```python
from build123d import *

# Parameters (mm, degrees)
SKETCH1_R           = 2.55
BOSS_EXTRUDE2_DEPTH = 10
SKETCH2_R           = 2.55
BOSS_EXTRUDE3_DEPTH = 2


with BuildPart() as part:
    # Sketch1 → Boss-Extrude2 (new body)
    with BuildSketch(Plane.XY):
        with BuildLine():
            ThreePointArc((18.024150889, 186.79103775), (10.644862344, 190.724335457), (2.347067513, 191.759386777))
            ThreePointArc((2.347067513, 191.759386777), (0, 191.690468331), (-2.347067513, 191.759386777))
            ThreePointArc((-2.347067513, 191.759386777), (-10.644862344, 190.724335457), (-18.024150889, 186.79103775))
            ThreePointArc((-18.024150889, 186.79103775), (-28.284271247, 194.215728749), (-35.708962247, 204.475849108))
            ThreePointArc((-35.708962247, 204.475849108), (-31.77566454, 211.855137653), (-30.74061322, 220.152932484))
            ThreePointArc((-30.74061322, 220.152932484), (-30.809531665, 222.499999997), (-30.74061322, 224.84706751))
            ThreePointArc((-30.74061322, 224.84706751), (-31.77566454, 233.14486234), (-35.708962247, 240.524150885))
            ThreePointArc((-35.708962247, 240.524150885), (-28.284271247, 250.784271244), (-18.024150889, 258.208962244))
            ThreePointArc((-18.024150889, 258.208962244), (-10.644862344, 254.275664537), (-2.347067513, 253.240613217))
            ThreePointArc((-2.347067513, 253.240613217), (0, 253.309531662), (2.347067513, 253.240613217))
            ThreePointArc((2.347067513, 253.240613217), (10.644862344, 254.275664537), (18.024150889, 258.208962244))
            ThreePointArc((18.024150889, 258.208962244), (28.284271247, 250.784271244), (35.708962247, 240.524150885))
            ThreePointArc((35.708962247, 240.524150885), (31.77566454, 233.14486234), (30.74061322, 224.84706751))
            ThreePointArc((30.74061322, 224.84706751), (30.809531665, 222.499999997), (30.74061322, 220.152932484))
            ThreePointArc((30.74061322, 220.152932484), (31.77566454, 211.855137653), (35.708962247, 204.475849108))
            ThreePointArc((35.708962247, 204.475849108), (28.284271247, 194.215728749), (18.024150889, 186.79103775))
        make_face()
        with Locations((-22.627416998, 245.127416995)):
            Circle(SKETCH1_R, mode=Mode.SUBTRACT)
        with Locations((-22.627416998, 199.872582999)):
            Circle(SKETCH1_R, mode=Mode.SUBTRACT)
        with Locations((22.627416998, 199.872582999)):
            Circle(SKETCH1_R, mode=Mode.SUBTRACT)
        with Locations((22.627416998, 245.127416995)):
            Circle(SKETCH1_R, mode=Mode.SUBTRACT)
        with BuildLine():
            Line((-15, 218.499999997), (-15, 199.25))
            Line((-15, 199.25), (15, 199.25))
            Line((15, 199.25), (15, 218.499999997))
            ThreePointArc((15, 218.499999997), (19, 222.499999997), (15, 226.499999997))
            Line((15, 226.499999997), (15, 245.749999994))
            Line((15, 245.749999994), (-15, 245.749999994))
            Line((-15, 245.749999994), (-15, 226.499999997))
            ThreePointArc((-15, 226.499999997), (-19, 222.499999997), (-15, 218.499999997))
        make_face(mode=Mode.SUBTRACT)
    extrude(amount=BOSS_EXTRUDE2_DEPTH)

    # Sketch2 → Boss-Extrude3 (add)
    with BuildSketch(Plane.XY.offset(10)):
        with BuildLine():
            ThreePointArc((18.024150889, 186.79103775), (28.284271247, 194.215728749), (35.708962247, 204.475849108))
            ThreePointArc((35.708962247, 204.475849108), (31.77566454, 211.855137653), (30.74061322, 220.152932484))
            ThreePointArc((30.74061322, 220.152932484), (30.809531665, 222.499999997), (30.74061322, 224.84706751))
            ThreePointArc((30.74061322, 224.84706751), (31.77566454, 233.14486234), (35.708962247, 240.524150885))
            ThreePointArc((35.708962247, 240.524150885), (28.284271247, 250.784271244), (18.024150889, 258.208962244))
            ThreePointArc((18.024150889, 258.208962244), (10.644862344, 254.275664537), (2.347067513, 253.240613217))
            ThreePointArc((2.347067513, 253.240613217), (0, 253.309531662), (-2.347067513, 253.240613217))
            ThreePointArc((-2.347067513, 253.240613217), (-10.644862344, 254.275664537), (-18.024150889, 258.208962244))
            ThreePointArc((-18.024150889, 258.208962244), (-28.284271247, 250.784271244), (-35.708962247, 240.524150885))
            ThreePointArc((-35.708962247, 240.524150885), (-31.77566454, 233.14486234), (-30.74061322, 224.84706751))
            ThreePointArc((-30.74061322, 224.84706751), (-30.809531665, 222.499999997), (-30.74061322, 220.152932484))
            ThreePointArc((-30.74061322, 220.152932484), (-31.77566454, 211.855137653), (-35.708962247, 204.475849108))
            ThreePointArc((-35.708962247, 204.475849108), (-28.284271247, 194.215728749), (-18.024150889, 186.79103775))
            ThreePointArc((-18.024150889, 186.79103775), (-10.644862344, 190.724335457), (-2.347067513, 191.759386777))
            ThreePointArc((-2.347067513, 191.759386777), (0, 191.690468331), (2.347067513, 191.759386777))
            ThreePointArc((2.347067513, 191.759386777), (10.644862344, 190.724335457), (18.024150889, 186.79103775))
        make_face()
        with Locations((-22.627416998, 245.127416995)):
            Circle(SKETCH2_R, mode=Mode.SUBTRACT)
        with Locations((-22.627416998, 199.872582999)):
            Circle(SKETCH2_R, mode=Mode.SUBTRACT)
        with Locations((22.627416998, 199.872582999)):
            Circle(SKETCH2_R, mode=Mode.SUBTRACT)
        with Locations((22.627416998, 245.127416995)):
            Circle(SKETCH2_R, mode=Mode.SUBTRACT)
        with BuildLine():
            Line((-15, 245.749999994), (-15, 226.499999997))
            ThreePointArc((-15, 226.499999997), (-19, 222.499999997), (-15, 218.499999997))
            Line((-15, 218.499999997), (15, 218.499999997))
            ThreePointArc((15, 218.499999997), (19, 222.499999997), (15, 226.499999997))
            Line((15, 226.499999997), (15, 245.749999994))
            Line((15, 245.749999994), (-15, 245.749999994))
        make_face(mode=Mode.SUBTRACT)
    extrude(amount=BOSS_EXTRUDE3_DEPTH)


solid = part.part
```
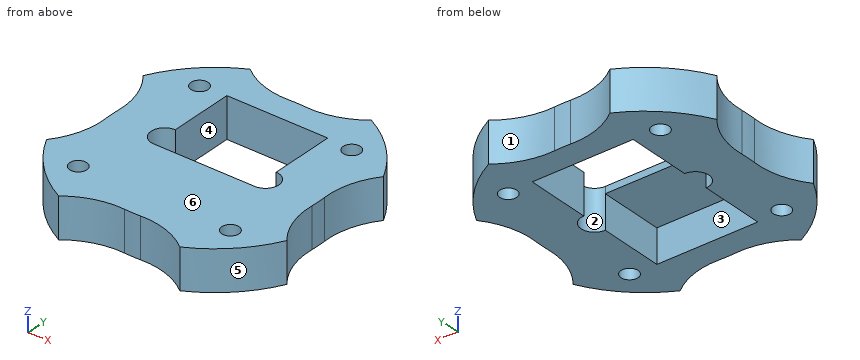
Input: part model. Units: mm. Frame: model coordinates. Face numbers are marked on the shaded views. A direction names the side the tool comes from. Coordinates: 2 decimals unless noted, no trailing zeros. Write each loop counter-clockwise with the first axis right and the second up, starting at its lowest first coordinate (ties: lowest second). Pieces come first, ordered by that corner, then holes. Notation, with made-up numbers: (31.25, -0.5) -> (63.25, -0.5) arc R32 cw to (63.25, 34.5) -> close; hole circle Ø9 at (80.25, 75.5). An arc over 180 degrees is marked (long way). Answer as a JSON object with one key per item and string values.
1. Section B-B on x = -8.5. Return the cut outline in (y, z), then the cut area to 3 significant figures.
Result set:
{"outline": "(191.29, 0) -> (199.25, 0) -> (199.25, 10) -> (218.5, 10) -> (218.5, 12) -> (191.29, 12) -> close; (245.75, 0) -> (253.71, 0) -> (253.71, 12) -> (245.75, 12) -> close", "area": "229 mm2"}
2. Mould query, pull axis X, two halves, no side actions, for the marked faces 4, 5 and 6. Classes: released by +X, released by -X, zero draft, split by the parting line, or undercut.
Result set:
{"face 4": "undercut", "face 5": "released by +X", "face 6": "zero draft"}
3. First-contact query: P1, Ø1.5, axis at x = 21.5, z = 3.5, coming from the -Y side; P2, Ø6, axis at x = -3.5, z = 4, coming from the -Y side; P3, Ø5, axis at x = -16, z = 8, coming from the -Y side. Flat tips, straight axial feed; report the tip coordinate or a pass-through.
Result set:
{"P1": "stops at y = 188.3", "P2": "stops at y = 191.63", "P3": "stops at y = 186.79"}
4. Access query for the marked faces 1, 2 and 3. Directions: +Z, -Z, +X, -X, +Y, -Y. A direction counts if a zero-diameter tool reaches every point of the face in a straight line with its end or side. Return the directions, or none.
Result set:
{"face 1": "+Z, -Z, +Y", "face 2": "+Z, -Z", "face 3": "-Z"}
5. Section A-A on y = 222.5. Return the cut outline in (x, z), then the cut area to 3 significant figures.
Result set:
{"outline": "(-30.81, 0) -> (-19, 0) -> (-19, 12) -> (-30.81, 12) -> close; (19, 0) -> (30.81, 0) -> (30.81, 12) -> (19, 12) -> close", "area": "283 mm2"}
6. Material intervals for line 1 (Y direction, x = -22.5, z = 1.75); line 2 (Y direction, x = 13, z = 9.75); line 3 (X direction, y = 237.5, z = 9.5), sorted ascending. Write a range as from..to.
Result set:
{"line 1": "y = 189.43..197.33, 202.42..242.58, 247.67..255.57", "line 2": "y = 189.83..199.25, 245.75..255.17", "line 3": "x = -33.67..-15, 15..33.67"}
7. Section D-D on y = 213. Return the cut outline in (x, z).
Result set:
{"outline": "(-31.45, 0) -> (-15, 0) -> (-15, 10) -> (15, 10) -> (15, 0) -> (31.45, 0) -> (31.45, 12) -> (-31.45, 12) -> close"}
8. Section C-C on z = 11. Return the cut outline in (x, y).
Result set:
{"outline": "(-35.71, 204.48) arc R40 ccw to (-18.02, 186.79) arc R23 cw to (-2.35, 191.76) arc R40 ccw to (2.35, 191.76) arc R23 cw to (18.02, 186.79) arc R40 ccw to (35.71, 204.48) arc R23 cw to (30.74, 220.15) arc R40 ccw to (30.74, 224.85) arc R23 cw to (35.71, 240.52) arc R40 ccw to (18.02, 258.21) arc R23 cw to (2.35, 253.24) arc R40 ccw to (-2.35, 253.24) arc R23 cw to (-18.02, 258.21) arc R40 ccw to (-35.71, 240.52) arc R23 cw to (-30.74, 224.85) arc R40 ccw to (-30.74, 220.15) arc R23 cw to start; hole circle Ø5.1 at (-22.63, 199.87); hole circle Ø5.1 at (-22.63, 245.13); hole (-15, 218.5) -> (15, 218.5) arc R4 ccw to (15, 226.5) -> (15, 245.75) -> (-15, 245.75) -> (-15, 226.5) arc R4 ccw to start; hole circle Ø5.1 at (22.63, 199.87); hole circle Ø5.1 at (22.63, 245.13)"}
